```python
from build123d import *

# Parameters (mm, degrees)
F0_W     = 42
F0_H     = 42
F0_R     = 11
F1_DEPTH = 40
F2_R     = 11
F3_DEPTH = 2
F4_R     = 2.5
F5_DEPTH = 20
F6_R     = 1.5
F7_DEPTH = 40.001


with BuildPart() as f1:
    # F0 (on Top) → F1 (new body)
    with BuildSketch(Plane.XY):
        Rectangle(F0_W, F0_H)
        Circle(F0_R, mode=Mode.SUBTRACT)
        Circle(F0_R)
    extrude(amount=F1_DEPTH)

    # F2 (on face) → F3 (join)
    with BuildSketch(Plane.XY.offset(40)):
        Circle(F2_R)
    extrude(amount=F3_DEPTH)

    # F4 (on face) → F5 (join)
    with BuildSketch(Plane.XY.offset(42)):
        Circle(F4_R)
    extrude(amount=F5_DEPTH)

    # F6 (on face) → F7 (cut, through all)
    with BuildSketch(Plane.XY.offset(40)):
        with Locations((-15.5, 15.5)):
            Circle(F6_R)
        with Locations((15.5, 15.5)):
            Circle(F6_R)
        with Locations((15.5, -15.5)):
            Circle(F6_R)
        with Locations((-15.5, -15.5)):
            Circle(F6_R)
    extrude(amount=-F7_DEPTH, mode=Mode.SUBTRACT)


solid = f1.part
```
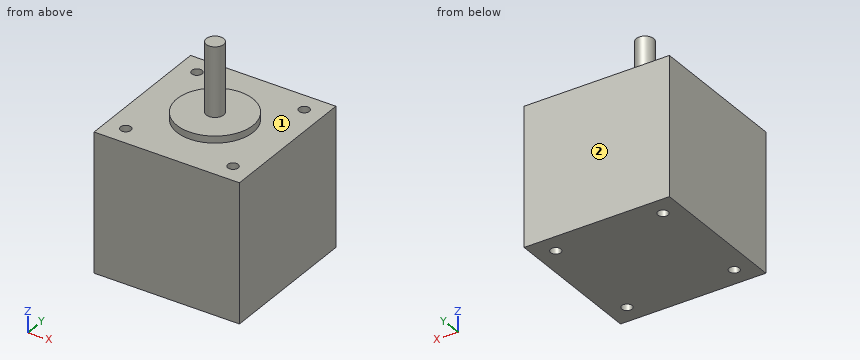
Geometry check sheet. Reference: the model listing, model coordinates, mm. Face numbers are marked on the shaded views. A direction names the side the tool comes from. Give positions to 0.01 mm unless a question says otherwise; leave off trailing zeros. Loops run counter-clockwise (first coordinate to the right, second up) from the corner with the lowest first, then second, coordinate; pieces in that order, holes last. Notation, with made-up numbers: M 0.5,-37 L 10.5,-37 A18 cw 10.5,-18 Z; hole C 46,50 d5. An arc over 180 degrees is marked long. Answer as CSV lines item,"result".
Item 1: Cross-section at A-A on y = -15.5. Record the cut outline in (x, z), and give its area (3 significant figures).
Values:
outline,"M -21,0 L -17,0 L -17,40 L -21,40 Z; M -14,0 L 14,0 L 14,40 L -14,40 Z; M 17,0 L 21,0 L 21,40 L 17,40 Z"
area,"1,440 mm²"
Item 2: Access from +Z, -Z, +X, -X, +Y, -Y to the whole of each face (thin tool, end or side, straight path). Record for the marked faces 1 and 2.
Values:
face 1,"+Z"
face 2,"+Z, -Z, +X, -X, +Y"
Item 3: Cross-section at C-C on z = 38.5. Record the cut outline in (x, y), and give its area (3 significant figures).
Values:
outline,"M -21,-21 L 21,-21 L 21,21 L -21,21 Z; hole C -15.5,-15.5 d3; hole C -15.5,15.5 d3; hole C 15.5,-15.5 d3; hole C 15.5,15.5 d3"
area,"1,740 mm²"
Item 4: Depth check by flat-ended pin: P1, Ø1.5, axis at x = -15.5, y = 7, coming from the -Z side; P2, Ø6.5, axis at x = -5.5, y = -2.5, coming from the +Z side; P3, Ø1.5, axis at x = -7.5, y = -10, coming from the +Z side; P4, Ø3, axis at x = -1.5, z = 46, coming from the +Y side. Enter the tip coordinate at first touch or a pass-through.
Values:
P1,"stops at z = 0"
P2,"stops at z = 42"
P3,"stops at z = 40"
P4,"stops at y = 2.5"
Item 5: Material ranges on line 1 (Y direction, x = 16, z = 23.5); line 2 (Y direction, x = -15.5, z = 15.5), recorded low to high.
Values:
line 1,"y = -21 to -16.91, -14.09 to 14.09, 16.91 to 21"
line 2,"y = -21 to -17, -14 to 14, 17 to 21"
Item 6: Cross-section at D-D on y = 0. Record the cut outline in (x, z), and give its area (3 significant figures).
Values:
outline,"M -21,0 L 21,0 L 21,40 L 11,40 L 11,42 L 2.5,42 L 2.5,62 L -2.5,62 L -2.5,42 L -11,42 L -11,40 L -21,40 Z"
area,"1,820 mm²"
